Source: CAD feature listing. Evaluate the final solid. Frame: model axes, mm. Face numbers are marked on the shaded views. Give positions to 0.01 mm unless a question says otherwise; leave off trailing zeros. Order: outer loops, then holes, each group sorted by start corner. A loop starts at its lowest first (then second) coordinate and runs counter-clockwise, first axis right, second up. Notation, with made-up numbers: M 12.25,24.5 L 58.25,24.5 A19 ccw 58.25,54.5 Z; hole C 73.5,29.25 d5. An arc over 180 degrees is marked long. Return JSON: item names as keys, results as strings.
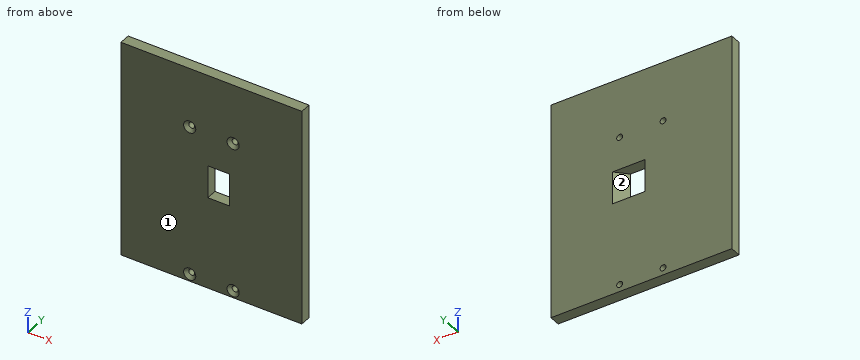
from build123d import *

# Parameters (mm, degrees)
F0_W           = 100
F0_H           = 120
F0_W_2         = 12
F0_H_2         = 18
F1_DEPTH       = 3
F2_SIZE        = 5.99999
F4_D           = 3.3
F4_CSINK_D     = 6.72
F4_CSINK_ANGLE = 90


# Not quite as in the source:
# - a fillet or chamfer is up to 0.001 mm smaller than in the source, because OpenCascade refuses the exact size


with BuildPart() as f1:
    # F0 (on Front) → F1 (new body, symmetric)
    with BuildSketch(Plane.XZ):
        Rectangle(F0_W, F0_H)
        with Locations((4, 0)):
            Rectangle(F0_W_2, F0_H_2, mode=Mode.SUBTRACT)
    extrude(amount=F1_DEPTH, both=True)

    # F2 (size 6 in the source; OpenCascade refuses exactly that, so slightly less here)
    f2_edges = [f1.edges().sort_by_distance(p)[0] for p in [
        (10, 3, 0),
    ]]
    chamfer(f2_edges, length=F2_SIZE)

    # F4 (through all)
    with Locations(Plane.XZ.offset(3)):
        with Locations((-12, 27), (12, 27), (12, -56), (-12, -56)):
            CounterSinkHole(F4_D / 2, F4_CSINK_D / 2, counter_sink_angle=F4_CSINK_ANGLE)


solid = f1.part
1. Section query C-C (x = -12). Return loops of the section in (y, z).
Evaluation:
{"outline": "M -3,-60 L 3,-60 L 3,-57.65 L -1.29,-57.65 L -3,-59.36 Z; M -3,-52.64 L -1.29,-54.35 L 3,-54.35 L 3,25.35 L -1.29,25.35 L -3,23.64 Z; M -3,30.36 L -1.29,28.65 L 3,28.65 L 3,60 L -3,60 Z"}
2. Draft query along Z for the marked faces 1 and 2. Return one class per face: pulls with the +Z half, pulls with the -Z half, needs draft (parallel to the pull), parting line crosses it, or undercut.
Evaluation:
{"face 1": "needs draft", "face 2": "undercut"}
3. Ray query, probe 1 along Z at (x, y) = (12, 1.8); probe 2 along X at (y, z) = (0.35, -56); probe 3 along Z at (x, y) = (-12, 2). Return the intervals inside material, ascending.
Evaluation:
{"probe 1": "z = -60 to -57.65, -54.35 to -9, 9 to 25.35, 28.65 to 60", "probe 2": "x = -50 to -13.65, -10.35 to 10.35, 13.65 to 50", "probe 3": "z = -60 to -57.65, -54.35 to 25.35, 28.65 to 60"}
4. First-contact query: pin 1 (4.5 mm diameter, centred on x = -12, z = -56, fed in from -Y). Flat tip, straight axial feed; report the tip coordinate or a pass-through.
Evaluation:
{"pin 1": "stops at y = -1.89"}
5. Section query D-D (y = 1.75). Return loops of the section in (x, z), then the cut area to 3 significant figures.
Evaluation:
{"outline": "M -50,-60 L 50,-60 L 50,60 L -50,60 Z; hole C -12,-56 d3.3; hole C -12,27 d3.3; hole M -2,-9 L 14.75,-9 L 14.75,9 L -2,9 Z; hole C 12,-56 d3.3; hole C 12,27 d3.3", "area": "11,700 mm^2"}
6. Section query B-B (z = 27). Return loops of the section in (x, y).
Evaluation:
{"outline": "M -50,-3 L -15.36,-3 L -13.65,-1.29 L -13.65,3 L -50,3 Z; M -10.35,-1.29 L -8.64,-3 L 8.64,-3 L 10.35,-1.29 L 10.35,3 L -10.35,3 Z; M 13.65,-1.29 L 15.36,-3 L 50,-3 L 50,3 L 13.65,3 Z"}
7. Section query A-A (x = 1.5). Return loops of the section in (y, z).
Evaluation:
{"outline": "M -3,-60 L 3,-60 L 3,-9 L -3,-9 Z; M -3,9 L 3,9 L 3,60 L -3,60 Z"}
